from build123d import *

# Parameters (mm, degrees)
SKETCH1_R               = 2.5
BOSS_EXTRUDE1_DEPTH     = 5
CUT_EXTRUDE2_DEPTH      = 445.100213916
CUT_EXTRUDE2_DEPTH_BACK = 445.100213916


with BuildPart() as part:
    # Sketch1 → Boss-Extrude1 (new body)
    with BuildSketch(Plane(origin=(0, 0, 0), x_dir=(1, 0, 0), z_dir=(0, 1, 0))):
        with BuildLine():
            Line((50, 0), (150, 0))
            ThreePointArc((150, 0), (185.355339059, -14.644660941), (200, -50))
            Line((200, -50), (200, -60))
            Line((200, -60), (260, -60))
            Line((260, -60), (260, 0))
            Line((260, 0), (250, 0))
            ThreePointArc((250, 0), (214.644660941, 14.644660941), (200, 50))
            Line((200, 50), (200, 250))
            ThreePointArc((200, 250), (214.644660941, 285.355339059), (250, 300))
            Line((250, 300), (260, 300))
            Line((260, 300), (260, 360))
            Line((260, 360), (200, 360))
            Line((200, 360), (200, 350))
            ThreePointArc((200, 350), (185.355339059, 314.644660941), (150, 300))
            Line((150, 300), (50, 300))
            ThreePointArc((50, 300), (14.644660941, 314.644660941), (0, 350))
            Line((0, 350), (0, 360))
            Line((0, 360), (-60, 360))
            Line((-60, 360), (-60, 300))
            Line((-60, 300), (-50, 300))
            ThreePointArc((-50, 300), (-14.644660941, 285.355339059), (0, 250))
            Line((0, 250), (0, 50))
            ThreePointArc((0, 50), (-14.644660941, 14.644660941), (-50, 0))
            Line((-50, 0), (-60, 0))
            Line((-60, 0), (-60, -60))
            Line((-60, -60), (0, -60))
            Line((0, -60), (0, -50))
            ThreePointArc((0, -50), (14.644660941, -14.644660941), (50, 0))
        make_face()
        with Locations(Location((20, 230, 0), (0, 0, 270))):
            Circle(SKETCH1_R, mode=Mode.SUBTRACT)
        with Locations(Location((20, 70, 0), (0, 0, 270))):
            Circle(SKETCH1_R, mode=Mode.SUBTRACT)
        with Locations(Location((180, 70, 0), (0, 0, 270))):
            Circle(SKETCH1_R, mode=Mode.SUBTRACT)
        with Locations(Location((180, 230, 0), (0, 0, 270))):
            Circle(SKETCH1_R, mode=Mode.SUBTRACT)
        with Locations(Location((-55, -30, 0), (0, 0, 270))):
            Circle(SKETCH1_R, mode=Mode.SUBTRACT)
        with Locations(Location((-5, -30, 0), (0, 0, 270))):
            Circle(SKETCH1_R, mode=Mode.SUBTRACT)
        with Locations(Location((-55, 330, 0), (0, 0, 270))):
            Circle(SKETCH1_R, mode=Mode.SUBTRACT)
        with Locations(Location((-5, 330, 0), (0, 0, 270))):
            Circle(SKETCH1_R, mode=Mode.SUBTRACT)
        with Locations(Location((205, 330, 0), (0, 0, 270))):
            Circle(SKETCH1_R, mode=Mode.SUBTRACT)
        with Locations(Location((255, 330, 0), (0, 0, 270))):
            Circle(SKETCH1_R, mode=Mode.SUBTRACT)
        with Locations(Location((205, -30, 0), (0, 0, 270))):
            Circle(SKETCH1_R, mode=Mode.SUBTRACT)
        with Locations(Location((255, -30, 0), (0, 0, 270))):
            Circle(SKETCH1_R, mode=Mode.SUBTRACT)
        with Locations(Location((100, 170, 0), (0, 0, 270))):
            Circle(SKETCH1_R, mode=Mode.SUBTRACT)
        with Locations(Location((120, 150, 0), (0, 0, 270))):
            Circle(SKETCH1_R, mode=Mode.SUBTRACT)
        with Locations(Location((80, 150, 0), (0, 0, 270))):
            Circle(SKETCH1_R, mode=Mode.SUBTRACT)
        with Locations(Location((100, 130, 0), (0, 0, 270))):
            Circle(SKETCH1_R, mode=Mode.SUBTRACT)
    extrude(amount=BOSS_EXTRUDE1_DEPTH)

    # Sketch3 → Cut-Extrude2 (cut, two sides: drawn at the far end of the back side and taken through both)
    with BuildSketch(Plane(origin=(0, 5, 0), x_dir=(1, 0, 0), z_dir=(0, 1, 0)).offset(-CUT_EXTRUDE2_DEPTH_BACK)):
        with BuildLine():
            Line((110, -806.241169496), (110, 0))
            ThreePointArc((110, 0), (100, 10), (90, 0))
            Line((90, 0), (90, -806.241169496))
            Line((90, -806.241169496), (90, -2418.723508487))
            Line((90, -2418.723508487), (110, -2418.723508487))
            Line((110, -2418.723508487), (110, -806.241169496))
        make_face()
    extrude(amount=CUT_EXTRUDE2_DEPTH + CUT_EXTRUDE2_DEPTH_BACK, mode=Mode.SUBTRACT)


solid = part.part
Work out the finished part from the listing and answer in its coordinate system (mm). A direction names the side the tool comes from. Round coordinates to 2 decimals unless told otherwise and drop trailing zeros. Order: outer loops, then holes, each group sorted by start corner. A loop starts at its lowest first (then second) coordinate and runs counter-clockwise, first axis right, second up. Notation, with made-up numbers: M -10,50 L 24,50 A26 ccw 24,68 Z; hole C -26,49.5 d7. An arc over 180 degrees is marked long. Put each result on its own line as item: value. Start each with the question number.
Q1. For a pull along Z with two mould halves and no side action, classify faces 1 (the cylindrical face through (184.964, 2.465, 14.258)), 2 (the cylindrical face through (15.036, 2.465, -314.258)), 3 (the cylindrical face through (-14.258, 2.465, -15.036)), 4 (the flat face through (98, 0, -153)) as pulls with the +Z half, pulls with the -Z half, needs draft (parallel to the pull), parting line crosses it, or undercut.
Q2. A tool of negligible diameter and unlimited length cuts with its end or side. For faces 5 (the cylindrical face through (14.258, 2.465, 15.036)), 6 (the flat face through (98, 5, -153)), 7 (the cylindrical face through (-15.036, 2.465, -285.742)), 8 (the cylindrical face through (185.742, 2.465, -315.036)), 9 (the cylindrical face through (215.036, 2.465, -14.258)), from which of +Z, -Z, +X, -X, +Y, -Y can it reach the whole face along a straight path? Write none if from no direction.
Q3. Straight lines are drawn through the part: L1, parallel to X at y = 3.35, z = -70; L2, parallel to X at y = 1.25, z = -70.5; L3, parallel to Z at x = 178, y = 1.6. For each, find the intervals that lie inside material, in ascending order. Write a range as [from, to].
Q4. Section B-B, the plane y = 3.4 is taken. Give the number of separate pieces and of enclosed holes in the cut face, and give its area (3 significant figures).
Q5. Section C-C, the plane x = 69 is taken. Write down the section's boundary in (y, z).
Q6. Section A-A, the plane z = -309.5 is taken. Write down the section's boundary in (x, y), and give its area (3 significant figures).
Q7. Flat-ended cylindrical pins translate along their axes: pin 1 (1.5 mm diameter, centred on y = 1, z = -88.5, fed in from -X); pin 2 (1.5 mm diameter, centred on y = 1.5, z = -194, fed in from +X); pin 3 (2 mm diameter, centred on x = 151, y = 1.5, fed in from -Z). Find the tip coordinate at first contact, or state that the pin passes through.
Findings below:
1. face 1: pulls with the +Z half
1. face 2: pulls with the -Z half
1. face 3: undercut
1. face 4: needs draft
2. face 5: +Z, +Y, -Y
2. face 6: +Z, -Z, +X, -X, +Y
2. face 7: -X, +Y, -Y
2. face 8: -Z, +Y, -Y
2. face 9: +X, +Y, -Y
3. L1: x = [0, 17.5], [22.5, 177.5], [182.5, 200]
3. L2: x = [0, 17.55], [22.45, 177.55], [182.45, 200]
3. L3: z = [-308.58, -231.5], [-228.5, -71.5], [-68.5, 8.58]
4. separate pieces: 1
4. enclosed holes: 16
4. area: 78,200 mm^2
5. outline: M 0,-300 L 5,-300 L 5,0 L 0,0 Z
6. outline: M -60,0 L 20.68,0 L 20.68,5 L -60,5 Z; M 179.32,0 L 260,0 L 260,5 L 179.32,5 Z
6. area: 807 mm^2
7. pin 1: stops at x = 0
7. pin 2: stops at x = 200
7. pin 3: stops at z = -300.04
